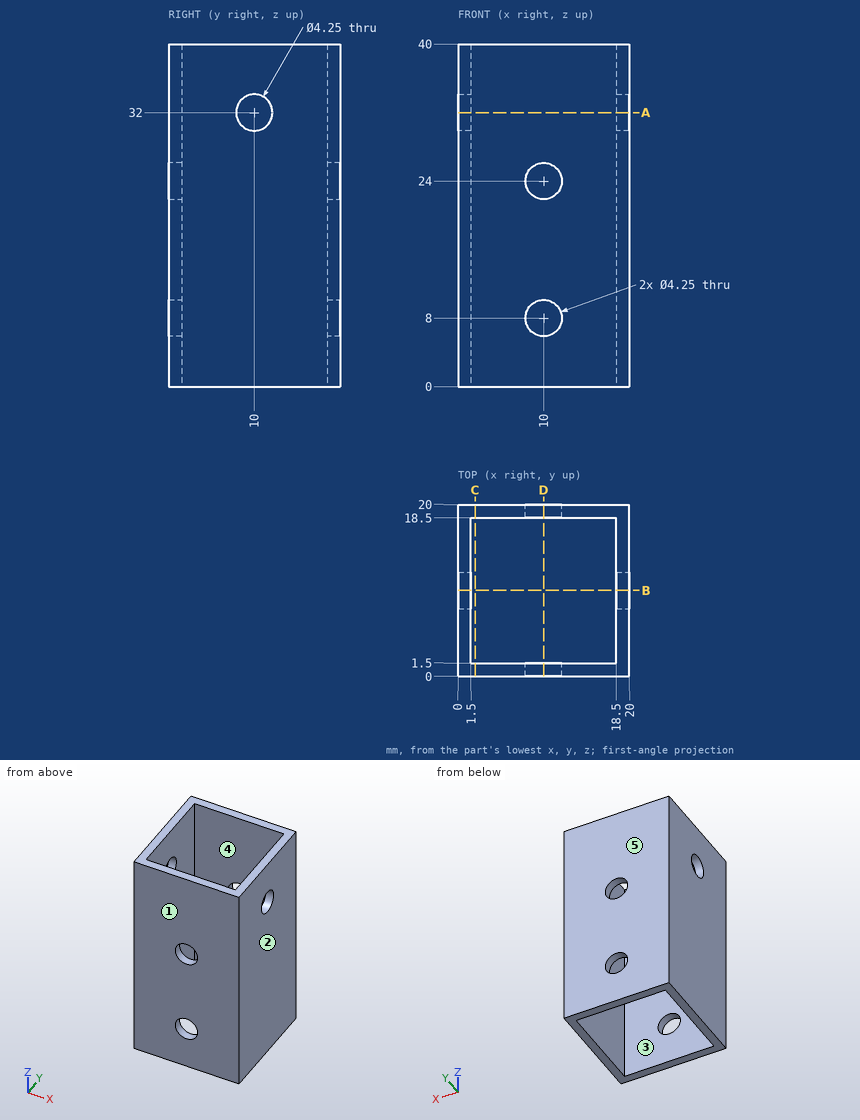
Check sheet for the drawn part. Datum: minimum x, y, z corner. Units: mm. A direction names the side the tool comes from. Round coordinates to 2 decimals unless told otherwise and drop trailing zeros. Order: outer loops, then holes, each group sorted by start corner. A loop starts at its lowest first (then second) coordinate and runs counter-clockwise, first axis right, second up. Notation, with made-up numbers: (30.25, 63) - (38.25, 63) arc R18 cw to (38.25, 89) - close; hole circle Ø10 at (35.25, 20). An arc over 180 degrees is marked (long way). Use a Markdown table: item, result. Add a question column.
(1) Sectioned sample at B-B, the plane y = 10. Enter the section's corners in (x, z) (3 decimals).
(2) Release check for a two-part mould opening along Y. For the marked faces 1, 2 and 3 record: pulls with the +Y half, pulls with the -Y half, needs draft (parallel to the pull), parting line crosses it, or undercut.
(3) Tool access check on the marked faces 4 and 5. Record the directions out of +Z, -Z, +X, -X, +Y, -Y that give a thin tool (end or side, any length) a straight path to the whole face; none if there is none.
(4) Material ranges on line 1 along Y through (x, z) = (2.5, 29.5); line 2 along X through (y, z) = (0.4, 24) (3 decimals), recorded low to high. Write a range as [from, to].
(5) Sectioned sample at A-A, the plane z = 32. Enter the section's corners in (x, y) (3 decimals).
(6) Sectioned sample at D-D, the plane x = 10. Enter the section's corners in (y, z) (3 decimals), and give its area (3 significant figures).
(7) Sectioned sample at C-C, the plane x = 2. Enter the section's corners in (y, z), and give its area (3 significant figures).
Answers below:
| question | item | result |
|---|---|---|
| 1 | outline | (0, 0) - (1.5, 0) - (1.5, 29.875) - (0, 29.875) - close; (0, 34.125) - (1.5, 34.125) - (1.5, 40) - (0, 40) - close; (18.5, 0) - (20, 0) - (20, 29.875) - (18.5, 29.875) - close; (18.5, 34.125) - (20, 34.125) - (20, 40) - (18.5, 40) - close |
| 2 | face 1 | pulls with the -Y half |
| 2 | face 2 | needs draft |
| 2 | face 3 | undercut |
| 3 | face 4 | +Z, -Z |
| 3 | face 5 | +Z, -Z, +X, -X, +Y |
| 4 | line 1 | [0, 1.5], [18.5, 20] |
| 4 | line 2 | [0, 7.875], [12.125, 20] |
| 5 | outline | (0, 0) - (20, 0) - (20, 7.875) - (18.5, 7.875) - (18.5, 1.5) - (1.5, 1.5) - (1.5, 7.875) - (0, 7.875) - close; (0, 12.125) - (1.5, 12.125) - (1.5, 18.5) - (18.5, 18.5) - (18.5, 12.125) - (20, 12.125) - (20, 20) - (0, 20) - close |
| 6 | outline | (0, 0) - (1.5, 0) - (1.5, 5.875) - (0, 5.875) - close; (0, 10.125) - (1.5, 10.125) - (1.5, 21.875) - (0, 21.875) - close; (0, 26.125) - (1.5, 26.125) - (1.5, 40) - (0, 40) - close; (18.5, 0) - (20, 0) - (20, 5.875) - (18.5, 5.875) - close; (18.5, 10.125) - (20, 10.125) - (20, 21.875) - (18.5, 21.875) - close; (18.5, 26.125) - (20, 26.125) - (20, 40) - (18.5, 40) - close |
| 6 | area | 94.5 mm² |
| 7 | outline | (0, 0) - (1.5, 0) - (1.5, 40) - (0, 40) - close; (18.5, 0) - (20, 0) - (20, 40) - (18.5, 40) - close |
| 7 | area | 120 mm² |
